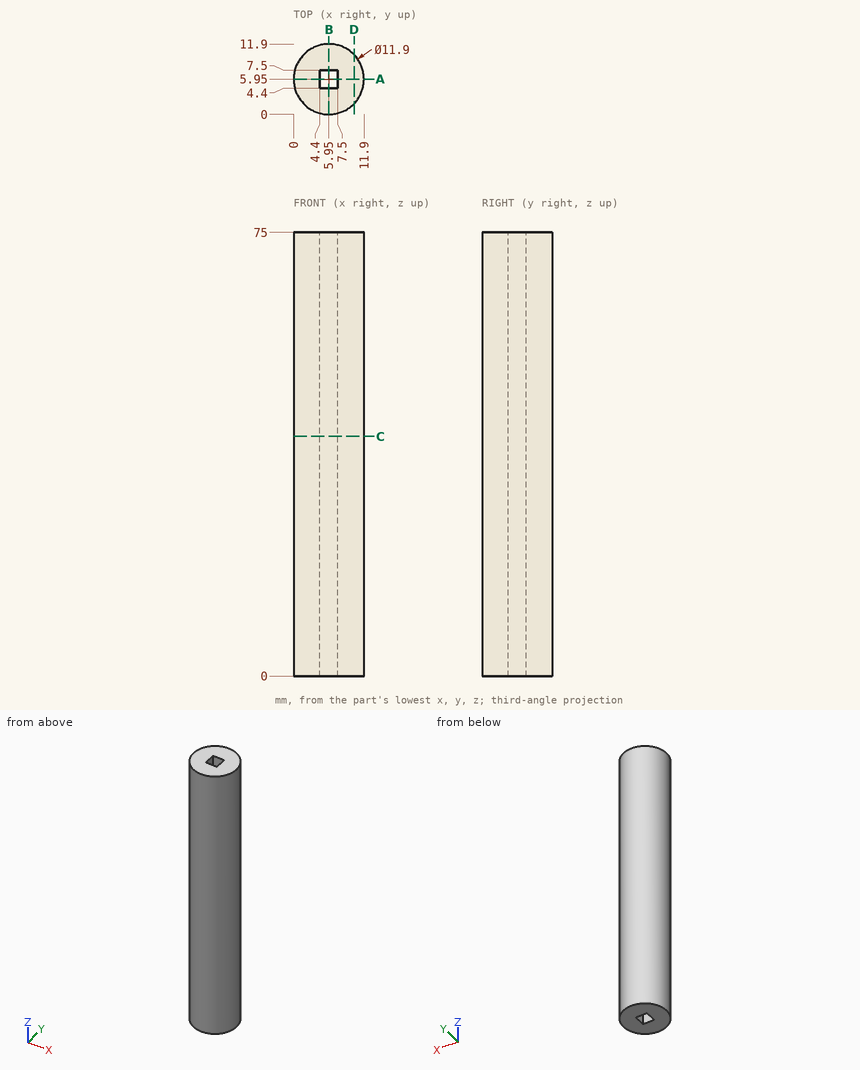
Drawing for the job (mm, zero at the part's lowest x, y, z). Round coordinates to 2 decimals unless told otherwise and drop trailing zeros. Write each loop counter-clockwise with the first axis right and the second up, starting at its lowest first coordinate (ties: lowest second). Pieces come first, ordered by that corner, then holes. Notation, with made-up numbers: (-18.75, -17) - (9.25, -17) arc R27 ccw to (9.25, 6) - close; hole circle Ø9 at (-2.75, 29). An arc over 180 degrees is marked (long way). Write item = value, one per line. Start each with the question number.
Q1. Drop a flat-ended pin along its axis: pin 1 (2 mm diameter, centred on y = 1.5, z = 63.5, fed in from +X). Give the stop position or say it passes through.
Q2. Band-saw the part on A-A (y = 5.95). Give the cut face in (x, z), then the cut area to 3 significant figures.
Q3. Band-saw the part on C-C (z = 40.5). Give the cut face in (x, y), then the cut area to 3 significant figures.
Q4. Probe L1, parallel to X at y = 6.25, z = 36; L2, parallel to Y at x = 6, z = 70.5; L3, parallel to Y at x = 8.75, z = 34.5. List the from-to ranges inside material, lowest first. Write a range as from..to.
Q5. Band-saw the part on D-D (x = 10.25). Give the cut face in (y, z).
Answers below:
q1.pin_1 = 10.8
q2.outline = (0, 0) - (4.4, 0) - (4.4, 75) - (0, 75) - close; (7.5, 0) - (11.9, 0) - (11.9, 75) - (7.5, 75) - close
q2.area = 660 mm2
q3.outline = circle Ø11.9 at (5.95, 5.95); hole (4.4, 4.4) - (7.5, 4.4) - (7.5, 7.5) - (4.4, 7.5) - close
q3.area = 102 mm2
q4.L1 = 0.01..4.4, 7.5..11.89
q4.L2 = 0..4.4, 7.5..11.9
q4.L3 = 0.7..11.2
q5.outline = (1.84, 0) - (10.06, 0) - (10.06, 75) - (1.84, 75) - close
